Read the model definition and answer for the solid it produces. Units are mm, in the model's axes. Face numbers are marked on the shaded views. A direction names the side the tool comes from. Give positions to 0.01 mm unless a question says otherwise; leave off trailing zeros. Order: outer loops, then holes, each group sorted by start corner. A loop starts at its lowest first (then second) coordinate and runs counter-clockwise, first axis right, second up. Notation, with made-up numbers: M -26.5,9.25 L 18.5,9.25 A19 cw 18.5,36.25 Z; hole C -27,22 d6. An arc over 180 degrees is marked long. One line per item, written item: value.
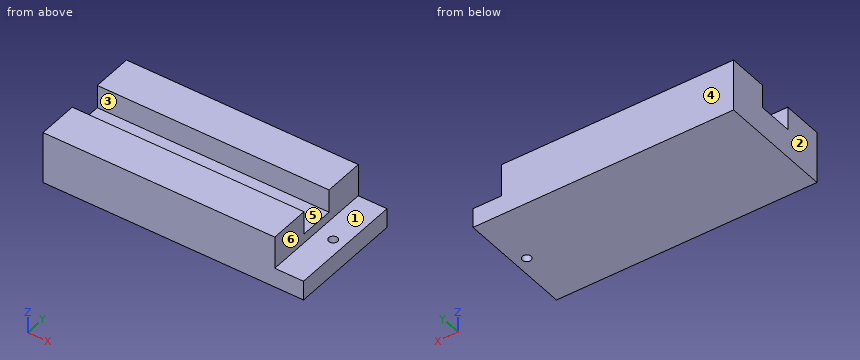
from build123d import *

# Parameters (mm, degrees)
F1_DEPTH = 63.5
F2_R     = 2.413
F3_DEPTH = 10.669
F4_W     = 19.05
F4_H     = 12.7
F5_DEPTH = 142.749


with BuildPart() as f1:
    # F0 (on Front) → F1 (new body)
    with BuildSketch(Plane.XZ):
        Polygon((-15.748, 28.448), (-142.748, 28.448), (-142.748, 0), (0, 0), (0, 10.668), (-15.748, 10.668), align=None)
    extrude(amount=F1_DEPTH)

    # F2 (on face) → F3 (cut, through all)
    with BuildSketch(Plane.XY.offset(10.668)):
        with Locations((-6.604, -31.75)):
            Circle(F2_R)
    extrude(amount=-F3_DEPTH, mode=Mode.SUBTRACT)

    # F4 (on face) → F5 (cut, through all)
    with BuildSketch(Plane(origin=(-142.748, 0, 0), x_dir=(0, -1, 0), z_dir=(-1, 0, 0))):
        with Locations((31.75, 22.098)):
            Rectangle(F4_W, F4_H)
    extrude(amount=-F5_DEPTH, mode=Mode.SUBTRACT)


solid = f1.part
1) Find section D-D, the plane y = -13.5. Write down the section's boundary in (x, z), plus the area to 3 significant figures.
Reported:
outline: M -142.75,0 L 0,0 L 0,10.67 L -15.75,10.67 L -15.75,28.45 L -142.75,28.45 Z
area: 3,780 mm^2
2) Find section C-C, the plane x = -31. Write down the section's boundary in (y, z) (3 decimals).
Reported:
outline: M -63.5,0 L 0,0 L 0,28.448 L -22.225,28.448 L -22.225,15.748 L -41.275,15.748 L -41.275,28.448 L -63.5,28.448 Z
3) Each of these flat-tipped pins is pushed along its axis until it touches: pin 1 Ø12 at (x, y) = (-100, -32) entering from +Z; pin 2 Ø8 at (x, y) = (-5, -29.5) entering from +Z. Where does it stop, or does it pass through?
Reported:
pin 1: stops at z = 15.75
pin 2: stops at z = 10.67
4) Which of the six approach directions +Z, -Z, +X, -X, +Y, -Y give full straight-line access (tool end or side, diameter ignored) to the marked faces 1 and 2?
Reported:
face 1: +Z, +X, +Y, -Y
face 2: +Z, -Z, -X, +Y, -Y
5) Find section B-B, the plane z = 17.5. Write down the section's boundary in (x, y) (3 decimals), plus the area to 3 significant figures.
Reported:
outline: M -142.748,-63.5 L -15.748,-63.5 L -15.748,-41.275 L -142.748,-41.275 Z; M -142.748,-22.225 L -15.748,-22.225 L -15.748,0 L -142.748,0 Z
area: 5,650 mm^2
6) Find section A-A, the plane y = -31.75. Write down the section's boundary in (x, z).
Reported:
outline: M -142.75,0 L -9.02,0 L -9.02,10.67 L -15.75,10.67 L -15.75,15.75 L -142.75,15.75 Z; M -4.19,0 L 0,0 L 0,10.67 L -4.19,10.67 Z
7) Consider probe 1 along Y at (x, z) = (-22, 21.75) (3 decimals); probe 2 along Z at (x, y) = (-12.5, -47); probe 3 along Z at (x, y) = (-74.5, -24). Determine where each line is inside the solid, lowest interval first.
Reported:
probe 1: y = -63.5 to -41.275, -22.225 to 0
probe 2: z = 0 to 10.67
probe 3: z = 0 to 15.75
8) Determine the mould class of the marked faces 3, 4, 5 and 6 for opening direction Y: +Y half, -Y half, draft (parallel to the pull), parting line (faces both ways), or undercut.
Reported:
face 3: undercut
face 4: +Y half
face 5: undercut
face 6: draft
